```python
from build123d import *

# Parameters (mm, degrees)
EXTRUDE_1_DEPTH     = 3
SKETCH_4_W          = 3
SKETCH_4_H          = 3.704951288
EXTRUDE_3_DEPTH     = 1
CUT_EXTRUDE_2_REACH = 25.05
SKETCH_6_R          = 0.5
CUT_EXTRUDE_1_DEPTH = 3


with BuildPart() as part:
    # 草图1 → 凸台-拉伸1 (new body)
    with BuildSketch(Plane.XY):
        with BuildLine():
            ThreePointArc((-4.975392322, 2.84990406), (-4.993840493, 2.675384142), (-5, 2.5))
            Line((-5, 2.5), (-5, -1.5))
            Line((-5, -1.5), (-5, -2.5))
            ThreePointArc((-5, -2.5), (-4.993840493, -2.675384142), (-4.975392322, -2.84990406))
            ThreePointArc((-4.975392322, -2.84990406), (-3.464823228, -3.464823228), (-2.84990406, -4.975392322))
            ThreePointArc((-2.84990406, -4.975392322), (-2.675384142, -4.993840493), (-2.5, -5))
            Line((-2.5, -5), (-1.5, -5))
            Line((-1.5, -5), (2.5, -5))
            ThreePointArc((2.5, -5), (2.675384142, -4.993840493), (2.84990406, -4.975392322))
            ThreePointArc((2.84990406, -4.975392322), (3.464823228, -3.464823228), (4.975392322, -2.84990406))
            ThreePointArc((4.975392322, -2.84990406), (4.993840493, -2.675384142), (5, -2.5))
            Line((5, -2.5), (5, 1.5))
            Line((5, 1.5), (5, 2.5))
            ThreePointArc((5, 2.5), (4.993840493, 2.675384142), (4.975392322, 2.84990406))
            ThreePointArc((4.975392322, 2.84990406), (3.464823228, 3.464823228), (2.84990406, 4.975392322))
            ThreePointArc((2.84990406, 4.975392322), (2.675384142, 4.993840493), (2.5, 5))
            Line((2.5, 5), (1.5, 5))
            Line((1.5, 5), (-2.5, 5))
            ThreePointArc((-2.5, 5), (-2.675384142, 4.993840493), (-2.84990406, 4.975392322))
            ThreePointArc((-2.84990406, 4.975392322), (-3.464823228, 3.464823228), (-4.975392322, 2.84990406))
        make_face()
        with BuildLine():
            ThreePointArc((-3.5, 2.5), (-3.207106781, 3.207106781), (-2.5, 3.5))
            Line((-2.5, 3.5), (2.5, 3.5))
            ThreePointArc((2.5, 3.5), (3.207106781, 3.207106781), (3.5, 2.5))
            Line((3.5, 2.5), (3.5, -2.5))
            ThreePointArc((3.5, -2.5), (3.207106781, -3.207106781), (2.5, -3.5))
            Line((2.5, -3.5), (-2.5, -3.5))
            ThreePointArc((-2.5, -3.5), (-3.207106781, -3.207106781), (-3.5, -2.5))
            Line((-3.5, -2.5), (-3.5, 2.5))
        make_face(mode=Mode.SUBTRACT)
        with BuildLine():
            Line((-5, -2.5), (-5, -1.5))
            ThreePointArc((-5, -1.5), (-5.161755993, -2.313202294), (-5.62239809, -3.00260191))
            Line((-5.62239809, -3.00260191), (-8.450825215, -5.831029035))
            Line((-8.450825215, -5.831029035), (-5.831029035, -8.450825215))
            Line((-5.831029035, -8.450825215), (-3.00260191, -5.62239809))
            ThreePointArc((-3.00260191, -5.62239809), (-2.313202294, -5.161755993), (-1.5, -5))
            Line((-1.5, -5), (-2.5, -5))
            ThreePointArc((-2.5, -5), (-2.675384142, -4.993840493), (-2.84990406, -4.975392322))
            ThreePointArc((-2.84990406, -4.975392322), (-4.267766953, -4.267766953), (-4.975392322, -2.84990406))
            ThreePointArc((-4.975392322, -2.84990406), (-4.993840493, -2.675384142), (-5, -2.5))
        make_face()
        with BuildLine():
            ThreePointArc((3.00260191, 5.62239809), (2.313202294, 5.161755993), (1.5, 5))
            Line((1.5, 5), (2.5, 5))
            ThreePointArc((2.5, 5), (2.675384142, 4.993840493), (2.84990406, 4.975392322))
            ThreePointArc((2.84990406, 4.975392322), (4.267766953, 4.267766953), (4.975392322, 2.84990406))
            ThreePointArc((4.975392322, 2.84990406), (4.993840493, 2.675384142), (5, 2.5))
            Line((5, 2.5), (5, 1.5))
            ThreePointArc((5, 1.5), (5.161755993, 2.313202294), (5.62239809, 3.00260191))
            Line((5.62239809, 3.00260191), (8.450825215, 5.831029035))
            Line((8.450825215, 5.831029035), (5.831029035, 8.450825215))
            Line((5.831029035, 8.450825215), (3.00260191, 5.62239809))
        make_face()
    extrude(amount=EXTRUDE_1_DEPTH)

    # 草图4 → 凸台-拉伸3 (add)
    with BuildSketch(Plane(origin=(-7.140927125, -7.140927125, 0), x_dir=(0, 0, 1), z_dir=(-0.707106781, -0.707106781, 0))):
        with Locations((1.5, 0)):
            Rectangle(SKETCH_4_W, SKETCH_4_H)
    extrude(amount=EXTRUDE_3_DEPTH)

    # 草图6 → 切除-拉伸2 (cut, up to next)
    with BuildSketch(Plane(origin=(7.140927125, 7.140927125, 0), x_dir=(0, 0, -1), z_dir=(0.707106781, 0.707106781, 0)), mode=Mode.PRIVATE) as cut_extrude_2_sk1:
        with Locations((-1.5, 0)):
            Circle(SKETCH_6_R)
    cut_extrude_2_tool1 = extrude(cut_extrude_2_sk1.sketch, amount=-CUT_EXTRUDE_2_REACH, mode=Mode.PRIVATE) & part.part
    add(cut_extrude_2_tool1.solids().sort_by_distance((7.140927, 7.140927, 1.5))[0], mode=Mode.SUBTRACT)

    # 草图5 → 切除-拉伸1 (cut)
    with BuildSketch(Plane.XY.offset(3)):
        with BuildLine():
            Line((-6.88210808, -6.175001298), (-5.467894517, -4.760787736))
            Line((-5.467894517, -4.760787736), (-6.424239217, -3.804443037))
            Line((-6.424239217, -3.804443037), (-9.157931996, -6.538135816))
            Line((-9.157931996, -6.538135816), (-7.848033901, -7.848033911))
            ThreePointArc((-7.848033901, -7.848033911), (-8.00695253, -6.640927128), (-6.88210808, -6.175001298))
        make_face()
        with BuildLine():
            Line((-3.804443037, -6.424239217), (-4.760787736, -5.467894517))
            Line((-4.760787736, -5.467894517), (-6.175001298, -6.88210808))
            ThreePointArc((-6.175001298, -6.88210808), (-6.149482263, -7.010400933), (-6.140927125, -7.140927125))
            ThreePointArc((-6.140927125, -7.140927125), (-6.758243689, -8.064806656), (-7.848033901, -7.848033911))
            Line((-7.848033901, -7.848033911), (-6.538135816, -9.157931996))
            Line((-6.538135816, -9.157931996), (-3.804443037, -6.424239217))
        make_face()
    extrude(amount=-CUT_EXTRUDE_1_DEPTH, mode=Mode.SUBTRACT)


solid = part.part
```
Geometry: final body of the model. Coordinates: model frame, mm. A direction names the side the tool comes from. Coordinates: 2 decimals unless noted, no trailing zeros. Order: outer loops, then holes, each group sorted by start corner. A loop starts at its lowest first (then second) coordinate and runs counter-clockwise, first axis right, second up. Notation, with made-up numbers: (-23, -38.75) - (-4, -38.75) arc R6 cw to (-4, -27.75) - close; hole circle Ø6 at (-28, 87.5). An arc over 180 degrees is marked (long way). Return JSON: item names as keys, results as strings. Group by question number.
1. Material intervals for line 1 along Y through (x, z) = (-1.25, 1.2); line 2 along Y through (x, z) = (-2.25, 2.05), sorted ascending. Write a range as [from, to].
2. Set-up query: faces 1 (the face through (0, -3.5, 1)), 2 (the face through (5, -1, 1)), 3 (the face through (0, 5, 1)). Return all of +Z, -Z, +X, -X, +Y, -Y with unobstructed straight access to the full face (end or side cutting, diameter ignored); none if empty.
3. Pull-direction query (X, two-part tool) for faces 4 (the face through (-2.324, -5.166, 1.479)), 5 (the face through (6.05, 5.36, 1.61)), 6 (the face through (-5, 1, 1)); classes: pulls with the +X half, pulls with the -X half, needs draft (parallel to the pull), parting line crosses it, or undercut.
4. Pin query (flat end, axial travel): pin 1 (1 mm diameter, centred on y = -2.5, z = 2, fed in from -X); pin 2 (1.5 mm diameter, centred on y = 1, z = 2, fed in from -X); pin 3 (0.9 mm diameter, centred on x = -1, z = 1.5, fed in from +Y). Return the tip coordinate at first contact, or that it passes through.
5. Cut plane C-C (x = 3.25). Output: boundary loops of the cut face in (y, z).
6. Cut plane D-D (z = 2.55). Count the separate pieces of the cut face and the enclosed holes in it, plus the area to 3 significant figures.
7. Cut plane A-A (y = 0.5). Output: boundary loops of the cut face in (x, z), plus the area to 3 significant figures.
Resolved:
{
 "1": {"line 1": "y = [-5, -3.5], [3.5, 5]", "line 2": "y = [-5.14, -3.5], [3.5, 5]"},
 "2": {"face 1": "+Z, -Z", "face 2": "+Z, -Z, +X, -Y", "face 3": "+Z, -Z, -X, +Y"},
 "3": {"face 4": "pulls with the +X half", "face 5": "undercut", "face 6": "pulls with the -X half"},
 "4": {"pin 1": "stops at x = -5.62", "pin 2": "stops at x = -5", "pin 3": "stops at y = 5"},
 "5": {"outline": "(-3.72, 0) - (-3.16, 0) - (-3.16, 3) - (-3.72, 3) - close; (3.16, 0) - (3.72, 0) - (3.72, 3) - (3.16, 3) - close; (4.88, 0) - (5.87, 0) - (5.87, 3) - (4.88, 3) - close"},
 "6": {"separate pieces": "1", "enclosed holes": "3", "area": "63.9 mm²"},
 "7": {"outline": "(-5, 0) - (-3.5, 0) - (-3.5, 3) - (-5, 3) - close; (3.5, 0) - (5, 0) - (5, 3) - (3.5, 3) - close", "area": "9.00 mm²"}
}
